Autodesk Inventor part; units mm, degrees
ref_plane "YZ Plane" through (0, 0, 0) normal (1, 0, 0) x (0, 1, 0)
ref_plane "XZ Plane" through (0, 0, 0) normal (0, 1, 0) x (-1, 0, 0)
ref_plane "XY Plane" through (0, 0, 0) normal (0, 0, 1) x (1, 0, 0)
sketch "VersaHex Adapter Hole" plane through (0, 0, 0) normal (0, 0, 1) x (1, 0, 0)
  line L0 (-2.6931, -2.4859) -> (-0.0712, 2.0554)
  arc A0 (1.4952, 2.9597) -> (-0.0712, 2.0554) centre (4.1171, -3.3903) ccw
  line L1 (1.4952, 2.9597) -> (6.7391, 2.9597)
  arc A1 (8.3055, 2.0554) -> (6.7391, 2.9597) centre (4.1171, -3.3903) ccw
  line L2 (8.3055, 2.0554) -> (10.9274, -2.4859)
  arc A2 (10.9274, -4.2946) -> (10.9274, -2.4859) centre (4.1171, -3.3903) ccw
  line L3 (10.9274, -4.2946) -> (8.3055, -8.8359)
  arc A3 (6.7391, -9.7403) -> (8.3055, -8.8359) centre (4.1171, -3.3903) ccw
  line L4 (6.7391, -9.7403) -> (1.4952, -9.7403)
  arc A4 (-0.0712, -8.8359) -> (1.4952, -9.7403) centre (4.1171, -3.3903) ccw
  line L5 (-0.0712, -8.8359) -> (-2.6931, -4.2946)
  arc A5 (-2.6931, -2.4859) -> (-2.6931, -4.2946) centre (4.1171, -3.3903) ccw
  point P0 (3.8427, -3.1642)
  point P1 (0, 3.175)
  point P2 (0, -3.175)
  point P3 (0, 0)
sketch "Block2" plane through (0, 0, 0) normal (0, 0, 1) x (1, 0, 0)
  line L0 (30.4112, -18.6542) -> (33.0331, -14.1129)
  arc A0 (34.5995, -13.2085) -> (33.0331, -14.1129) centre (37.2214, -19.5585) ccw
  line L1 (34.5995, -13.2085) -> (39.8433, -13.2085)
  arc A1 (41.4097, -14.1129) -> (39.8433, -13.2085) centre (37.2214, -19.5585) ccw
  line L2 (41.4097, -14.1129) -> (44.0316, -18.6542)
  arc A2 (44.0316, -20.4629) -> (44.0316, -18.6542) centre (37.2214, -19.5585) ccw
  line L3 (44.0316, -20.4629) -> (41.4097, -25.0042)
  arc A3 (39.8433, -25.9085) -> (41.4097, -25.0042) centre (37.2214, -19.5585) ccw
  line L4 (39.8433, -25.9085) -> (34.5995, -25.9085)
  arc A4 (33.0331, -25.0042) -> (34.5995, -25.9085) centre (37.2214, -19.5585) ccw
  line L5 (33.0331, -25.0042) -> (30.4112, -20.4629)
  arc A5 (30.4112, -18.6542) -> (30.4112, -20.4629) centre (37.2214, -19.5585) ccw
  point P0 (37.2214, -19.5585)
sketch "Sketch1" plane through (0, 0, 0) normal (0, 0, 1) x (1, 0, 0)
  circle A0 centre (-20.6222, -11.9063) radius 2.1526
  circle A1 centre (20.6222, -11.9062) radius 2.1526
  circle A2 centre (0, 23.8125) radius 2.1526
  arc A3 (-24.0046, -8.5535) -> (-19.4099, -16.5119) centre (-20.6222, -11.9063) ccw
  arc A4 (19.4099, -16.5119) -> (24.0046, -8.5535) centre (20.6222, -11.9062) ccw
  arc A5 (4.5947, 25.0654) -> (-4.5947, 25.0654) centre (0, 23.8125) ccw
  arc A6 (19.4099, -16.5119) -> (-19.4099, -16.5119) centre (0, -90.2489) ccw
  arc A7 (-24.0046, -8.5535) -> (-4.5947, 25.0654) centre (-78.1579, 45.1245) ccw
  arc A8 (4.5947, 25.0654) -> (24.0046, -8.5535) centre (78.1579, 45.1245) ccw
  line L0 (-6.8102, 0.9044) -> (-4.1883, 5.4456)
  arc A9 (-2.6219, 6.35) -> (-4.1883, 5.4456) centre (0, 0) ccw
  line L1 (-2.6219, 6.35) -> (2.6219, 6.35)
  arc A10 (4.1883, 5.4456) -> (2.6219, 6.35) centre (0, 0) ccw
  line L2 (4.1883, 5.4456) -> (6.8102, 0.9044)
  arc A11 (6.8102, -0.9044) -> (6.8102, 0.9044) centre (0, 0) ccw
  line L3 (6.8102, -0.9044) -> (4.1883, -5.4456)
  arc A12 (2.6219, -6.35) -> (4.1883, -5.4456) centre (0, 0) ccw
  line L4 (2.6219, -6.35) -> (-2.6219, -6.35)
  arc A13 (-4.1883, -5.4456) -> (-2.6219, -6.35) centre (0, 0) ccw
  line L5 (-4.1883, -5.4456) -> (-6.8102, -0.9044)
  arc A14 (-6.8102, 0.9044) -> (-6.8102, -0.9044) centre (0, 0) ccw
  dimension "d5" = 9.525
  dimension "d6" = 9.525
  dimension "d7" = 9.525
extrude "Extrusion1" add sketch "Sketch1" along normal blind 1.5875
equation "\"BendRadius\" = Thickness"
equation "\"BendReliefWidth\" = Thickness"
equation "\"BendReliefDepth\" = 0.5 * Thickness"
equation "\"CornerReliefSize\" = 4 * Thickness"
equation "\"MinimumRemnant\" = 2 * Thickness"
equation "\"TransitionRadius\" = BendRadius"
equation "\"JacobiRadiusSize\" = BendRadius"
equation "\"GapSize\" = Thickness"
properties part number "flex_wheel_hub" material "Acetal Resin, White"
Model file for the job. Use its own axes, mm. A direction names the side the tool comes from. Give positions to 0.01 mm unless a question says otherwise; leave off trailing zeros. Loops run counter-clockwise (first coordinate to the right, second up) from the corner with the lowest first, then second, coordinate; pieces in that order, holes last. Notation, with made-up numbers: (-14.5, -35.75) - (17.5, -35.75) arc R30 cw to (17.5, 2.25) - close; hole circle Ø2 at (81.25, -12). An arc over 180 degrees is marked (long way). One line per item, written item: value. Start each with the question number.
1. Slice it at B-B (y = 4.5). List the corners of the cut face in (x, z).
2. Probe L1, parallel to Y at x = -1, z = 0.1; L2, parallel to X at y = -3, z = 0.1; L3, parallel to X at y = -10, z = 0.85. List the from-to ranges inside material, lowest first. Write a range as from..to.
3. Pin check, flat tip, straight feed: pin 1 (0.8 mm diameter, centred on x = -1, z = 1, fed in from +Y). Stop position of the tip, or through.
4. Pull direction X, two halves, no side cores. Call faces 3 (the cylindrical face through (-11.987, 7.238, 0.783)), 4 (the flat face through (-5.52, 3.14, 0.78)), 5 (the cylindrical face through (-0.087, 28.574, 0.783)): pulls with the +X half, pulls with the -X half, needs draft (parallel to the pull), parting line crosses it, or undercut.
5. Which spindle directions (+Z, -Z, +X, -X, +Y, -Y) get a long thin tool onto all of the face, cutting with end or side? Do faces 1 (the cylindrical face through (3.42, 5.96, 0.78)), 2 (the flat face through (-6, -4, 1.588)). Say none if no direction does.
6. Slice it at D-D (x = 22). List the corners of the cut face in (y, z), plus the area to 3 significant figures.
7. Slice it at A-A (x = 0). List the corners of the cut face in (y, z), plus the area to 3 significant figures.
8. Slice it at C-C (z = 0.6). Give the number of separate pieces and of enclosed holes in the cut face, plus the area to 3 significant figures.
Solution:
1. outline: (-13.63, 0) - (-4.73, 0) - (-4.73, 1.59) - (-13.63, 1.59) - close; (4.73, 0) - (13.63, 0) - (13.63, 1.59) - (4.73, 1.59) - close
2. L1: y = -14.01..-6.35, 6.35..21.91, 25.72..28.47
2. L2: x = -19.01..-5.6, 5.6..19.01
2. L3: x = -24.99..-21.62, -19.62..19.62, 21.62..24.99
3. pin 1: stops at y = 28.54
4. face 3: pulls with the -X half
4. face 4: undercut
4. face 5: parting line crosses it
5. face 1: +Z, -Z
5. face 2: +Z, +X, -X, +Y, -Y
6. outline: (-16.47, 0) - (-13.56, 0) - (-13.56, 1.59) - (-16.47, 1.59) - close; (-10.25, 0) - (-6.45, 0) - (-6.45, 1.59) - (-10.25, 1.59) - close
6. area: 10.6 mm^2
7. outline: (-14, 0) - (-6.35, 0) - (-6.35, 1.59) - (-14, 1.59) - close; (6.35, 0) - (21.66, 0) - (21.66, 1.59) - (6.35, 1.59) - close; (25.97, 0) - (28.57, 0) - (28.57, 1.59) - (25.97, 1.59) - close
7. area: 40.6 mm^2
8. separate pieces: 1
8. enclosed holes: 4
8. area: 1,000 mm^2
